Design review of the part built by this model. Coordinates are the model's own, in mm. Face numbers are marked on the shaded views. A direction names the side the tool comes from. Coordinates: 2 decimals unless noted, no trailing zeros. Loops run counter-clockwise (first coordinate to the right, second up) from the corner with the lowest first, then second, coordinate; pieces in that order, holes last. Notation, with made-up numbers: M 25.25,-17.5 L 81.25,-17.5 A21 ccw 81.25,-7.5 Z; hole C -20.5,-18 d4. An arc over 180 degrees is marked long. Write item = value, one per line. Start each with the question number.
from build123d import *

# Parameters (mm, degrees)
F1_DEPTH = 101.6
F2_W     = 101.6
F2_H     = 101.6
F3_DEPTH = 50.8
F4_W     = 50.8
F4_H     = 50.8
F5_DEPTH = 101.601


with BuildPart() as f1:
    # F0 (on Top) → F1 (new body)
    with BuildSketch(Plane.XY):
        Polygon((-101.6, 0), (0, 0), (0, 101.6), align=None)
    extrude(amount=F1_DEPTH)

    # F2 (on Top) → F3 (join)
    with BuildSketch(Plane.XY):
        with Locations((-50.8, 50.8)):
            Rectangle(F2_W, F2_H)
    extrude(amount=F3_DEPTH)

    # F4 (on face) → F5 (cut, through all)
    with BuildSketch(Plane(origin=(0, 0, 0), x_dir=(1, 0, 0), z_dir=(0, 0, -1))):
        with Locations((-76.2, -76.2)):
            Rectangle(F4_W, F4_H)
    extrude(amount=-F5_DEPTH, mode=Mode.SUBTRACT)


solid = f1.part
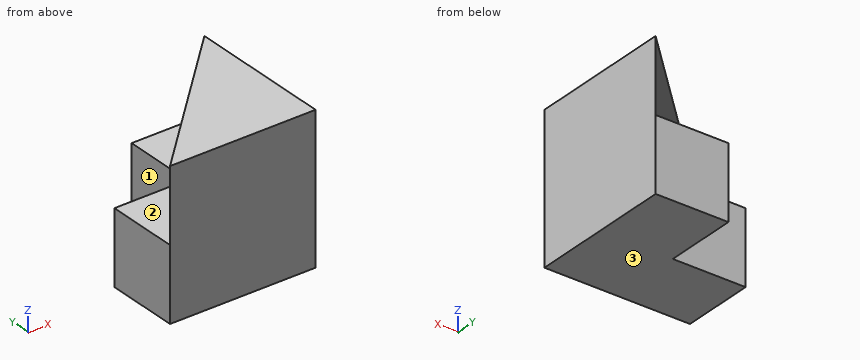
Q1. Add section B-B on x = -79.5. State the section outline as (y, z) points, plus the area to 3 significant figures.
Q2. Add section C-C on z = 76. State the section outline as (x, y) points.
Q3. For the marked faces 1, 2 and 3, list the 3-axis set-ups (+Z, -Z, +X, -X, +Y, -Y) from which the entire face can be reached by the end or side of a thin tool; tool diameter is ignored.
Q4. Clearance check with flat-ended pins moving along their axes: P1, Ø12, axis at x = -68, z = 43, coming from the +Y side; P2, Ø12, axis at x = -52, y = 87, coming from the +Z side; P3, Ø6, axis at y = 67.5, z = 81, coming from the -X side. State where each tip first meets the part, or that it passes through.
Q5. Add section A-A on z = 40.5. State the section outline as (x, y) points, plus the area to 3 significant figures.
Q6. To check wall thickness, follow line 1 (Y direction, x = -86, z = 22.5); line 2 (X direction, y = 80, z = 16). State the ranges of each line that lie inside material, in increasing order. Write a range as from..to.
Values follow:
q1.outline = M 0,0 L 50.8,0 L 50.8,50.8 L 22.1,50.8 L 22.1,101.6 L 0,101.6 Z
q1.area = 3,700 mm2
q2.outline = M -101.6,0 L 0,0 L 0,101.6 Z
q3.face_1 = +Z, -Z, -X, +Y
q3.face_2 = +Z, -X, +Y
q3.face_3 = -Z, +X, -X, +Y, -Y
q4.P1 = 50.8
q4.P2 = 50.8
q4.P3 = -37.1
q5.outline = M -101.6,0 L 0,0 L 0,101.6 L -50.8,101.6 L -50.8,50.8 L -101.6,50.8 Z
q5.area = 7,740 mm2
q6.line_1 = 0..50.8
q6.line_2 = -50.8..0
